Could you check a few things on this drawing? It's one solid part, dimensions in mm from its lowest x, y, z. Give positions to 0.01 mm unless a question says otherwise; leave off trailing zeros. Write each loop counter-clockwise with the first axis right and the second up, starting at its lowest first coordinate (ties: lowest second). Pieces come first, ordered by that corner, then holes. Notation, with made-up numbers: M 45,44.5 L 58,44.5 A11 ccw 58,51.5 Z; hole C 15,4 d3. An arc over 180 degrees is marked long. Use CSV: the item, a comma, the result in double quotes. Start each with the question number.
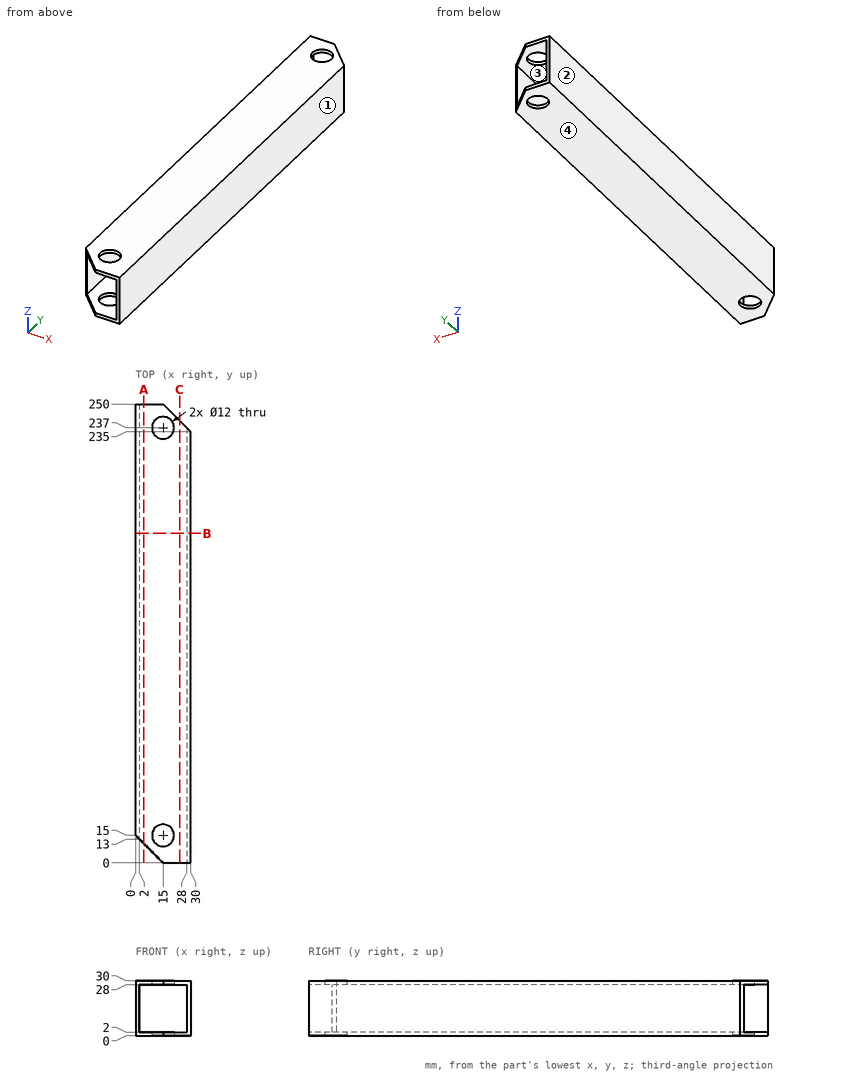
(1) I want a section at C-C (x = 24). Write out the boundary of the cut face in (y, z).
(2) I want a section at B-B (y = 179.5). Write out the boundary of the cut face in (x, z).
(3) Will this pin go through, and if not, where does the flat tip stop? pin 1 Ø11 at (x, y) = (15, 15) entering from +Z.
(4) I want a section at A-A (x = 4.5). Write out the boundary of the cut face in (y, z), and give its area (3 significant figures).
(5) Thinking about a two-plate mould opening in X: for the marked faces 1, 2, 3 and 4, which applies, released by +X, released by -X, zero draft, split by the parting line, or undercut?
(6) Please list where these lines run through material, in increasing order: L1, parallel to X at y = 73.5, z = 7; L2, parallel to X at y = 239.5, z = 10. Write a range as [from, to].
Geometry results:
1,outline,"M 0,0 L 241,0 L 241,2 L 0,2 Z; M 0,28 L 241,28 L 241,30 L 0,30 Z"
2,outline,"M 0,0 L 30,0 L 30,30 L 0,30 Z; hole M 2,2 L 28,2 L 28,28 L 2,28 Z"
3,pin 1,"passes through"
4,outline,"M 10.5,0 L 250,0 L 250,2 L 10.5,2 Z; M 10.5,28 L 250,28 L 250,30 L 10.5,30 Z"
4,area,"958 mm2"
5,face 1,"released by +X"
5,face 2,"released by -X"
5,face 3,"undercut"
5,face 4,"zero draft"
6,L1,"x = [0, 2], [28, 30]"
6,L2,"x = [0, 2]"
